from build123d import *

# Parameters (mm, degrees)
SKETCH3_W           = 92
SKETCH3_H           = 60
SKETCH3_W_2         = 76.5
SKETCH3_H_2         = 48
SKETCH3_R           = 2.25
SKETCH3_R_2         = 3
SKETCH3_W_3         = 56
SKETCH3_H_3         = 10.5
BOSS_EXTRUDE3_DEPTH = 20


with BuildPart() as part:
    # Sketch3 → Boss-Extrude3 (new body)
    # profile 1 of 2: a face of its own
    with BuildSketch(Plane.XY):
        with Locations((46, 30)):
            Rectangle(SKETCH3_W, SKETCH3_H)
        with Locations((46.25, 30)):
            Rectangle(SKETCH3_W_2, SKETCH3_H_2, mode=Mode.SUBTRACT)
    # profile 2 of 2: a face of its own
    with BuildSketch(Plane.XY):
        with Locations((46.25, 30)):
            Rectangle(SKETCH3_W_2, SKETCH3_H_2)
        with Locations((10.5, 51.5)):
            Circle(SKETCH3_R, mode=Mode.SUBTRACT)
        with Locations((10.5, 8.5)):
            Circle(SKETCH3_R, mode=Mode.SUBTRACT)
        with Locations((82, 8.5)):
            Circle(SKETCH3_R, mode=Mode.SUBTRACT)
        with Locations((82, 51.5)):
            Circle(SKETCH3_R, mode=Mode.SUBTRACT)
        with Locations((77, 30)):
            Circle(SKETCH3_R_2, mode=Mode.SUBTRACT)
        with Locations((55, 30)):
            Circle(SKETCH3_R_2, mode=Mode.SUBTRACT)
        with Locations((35, 30)):
            Circle(SKETCH3_R_2, mode=Mode.SUBTRACT)
        with Locations((15, 30)):
            Circle(SKETCH3_R_2, mode=Mode.SUBTRACT)
        with Locations((46.5, 13.75)):
            Rectangle(SKETCH3_W_3, SKETCH3_H_3, mode=Mode.SUBTRACT)
    extrude(amount=BOSS_EXTRUDE3_DEPTH)


solid = part.part
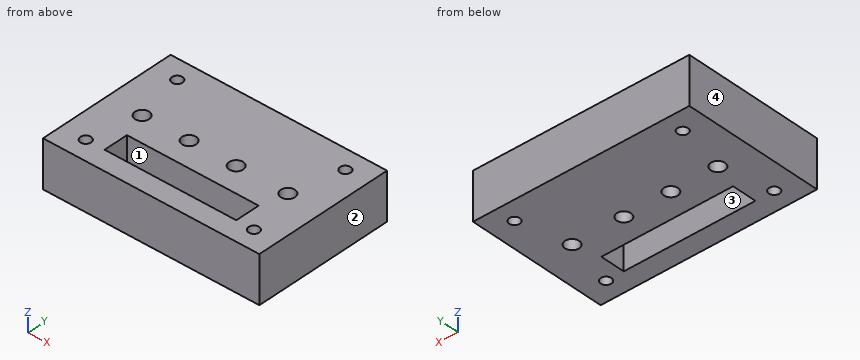
For this review, take the finished solid that the model builds, in its own axes (mm). Face numbers are marked on the shaded views. Give positions to 0.01 mm unless a question says otherwise; leave off trailing zeros. Order: outer loops, then holes, each group sorted by start corner. A loop starts at its lowest first (then second) coordinate and runs counter-clockwise, first axis right, second up. Notation, with made-up numbers: M 7,74 L 41,74 A23 cw 41,93 Z; hole C 19,43.5 d8. An arc over 180 degrees is marked long. Answer in a Markdown table with one row per item. Add a question column.
(1) Mouldability with a two-part tool opening along X and no side actions: class the marked faces 1, 2, 3 and 4 as +X half, -X half, draft (parallel to the pull), parting line (faces both ways), or undercut.
(2) Consider section B-B on x = 15. State the section outline as (y, z) points, and give its area (3 significant figures).
(3) For pin 1 (6 mm diameter, centred on y = 49, z = 11, fed in from -X); pin 2 (3.5 mm diameter, centred on x = 10.5, y = 8.5, fed in from +Z), all flat-tipped, find the tip position at first contact; note any pin that passes through.
(4) Consider section C-C on z = 16.25. Give the number of separate pieces and of enclosed holes in the cut face, and give its area (3 significant figures).
(5) Consider section A-A on x = 55. State the section outline as (y, z) points.
(6) Wall thickness on probe 1 along Y at (x, z) = (10.5, 4.25); probe 2 along Y at (x, z) = (39.5, 6.25); probe 3 along X at (y, z) = (16.5, 10.75): over which ranges is each line inside the solid? List them lowest first. Write a range as [from, to].
(7) Consider section D-D on y = 7.5. State the section outline as (x, z) points.
Evaluation:
| question | item | result |
|---|---|---|
| 1 | face 1 | undercut |
| 1 | face 2 | +X half |
| 1 | face 3 | undercut |
| 1 | face 4 | -X half |
| 2 | outline | M 0,0 L 27,0 L 27,20 L 0,20 Z; M 33,0 L 60,0 L 60,20 L 33,20 Z |
| 2 | area | 1,080 mm^2 |
| 3 | pin 1 | stops at x = 0 |
| 3 | pin 2 | passes through |
| 4 | separate pieces | 1 |
| 4 | enclosed holes | 9 |
| 4 | area | 4,760 mm^2 |
| 5 | outline | M 0,0 L 8.5,0 L 8.5,20 L 0,20 Z; M 19,0 L 27,0 L 27,20 L 19,20 Z; M 33,0 L 60,0 L 60,20 L 33,20 Z |
| 6 | probe 1 | y = [0, 6.25], [10.75, 49.25], [53.75, 60] |
| 6 | probe 2 | y = [0, 8.5], [19, 60] |
| 6 | probe 3 | x = [0, 18.5], [74.5, 92] |
| 7 | outline | M 0,0 L 8.48,0 L 8.48,20 L 0,20 Z; M 12.52,0 L 79.98,0 L 79.98,20 L 12.52,20 Z; M 84.02,0 L 92,0 L 92,20 L 84.02,20 Z |
